For this review, take the finished solid that the model builds, in its own axes (mm). Face numbers are marked on the shaded views. A direction names the side the tool comes from. Give positions to 0.01 mm unless a question says otherwise; leave off trailing zeros. Write each loop counter-clockwise with the first axis right and the second up, starting at its lowest first coordinate (ties: lowest second). Pieces come first, ordered by that corner, then holes. Notation, with made-up numbers: M -20,1 L -10,1 A27 cw -10,29 Z; hole C 59,1 d7. An arc over 180 degrees is marked long. Write item = value, one per line.
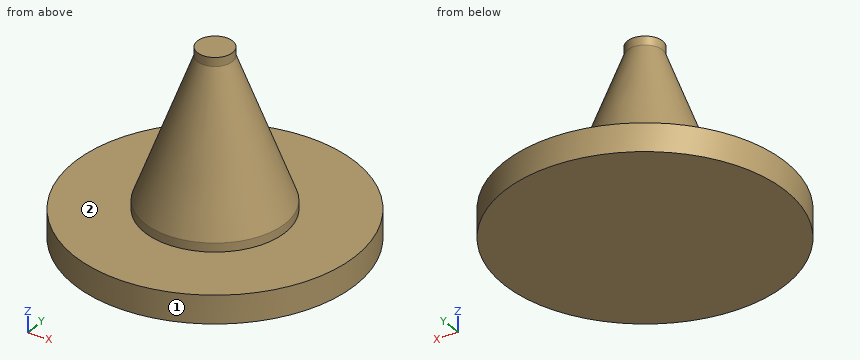
Autodesk Inventor part; units mm, degrees
ref_plane "YZ Plane" through (0, 0, 0) normal (1, 0, 0) x (0, 1, 0)
ref_plane "XZ Plane" through (0, 0, 0) normal (0, 1, 0) x (-1, 0, 0)
ref_plane "XY Plane" through (0, 0, 0) normal (0, 0, 1) x (1, 0, 0)
sketch "Sketch1" plane through (0, 0, 0) normal (0, 0, 1) x (1, 0, 0)
  circle A0 centre (0, 0) radius 12.7
  dimension "d0" = 25.4
extrude "Extrusion1" add sketch "Sketch1" along normal blind 1.5875
ref_plane "Work Plane1" through (0, 0, 26.9875) normal (0, 0, 1) x (1, 0, 0)
sketch "Sketch2" plane through (0, 0, 26.9875) normal (0, 0, 1) x (1, 0, 0)
  circle A0 centre (0, 0) radius 3.175
  dimension "d4" = 6.35
extrude "Extrusion2" add sketch "Sketch2" along normal blind 1.5875
loft "Loft1" add section 1 edges at (-12.7, 0, 1.5875) section 2 edges at (-3.175, 0, 26.9875)
sketch "Sketch3" plane through (0, 0, 0) normal (0, 0, -1) x (-1, 0, 0)
  circle A0 centre (0, 0) radius 25.4
  dimension "d11" = 50.8
extrude "Extrusion3" add sketch "Sketch3" along normal blind 5.08
sketch "Sketch5" plane through (0, 0, -5.08) normal (0, 0, -1) x (-1, 0, 0)
  point P0 (0, 0)
properties part number "Aerospike base"
1. We need section B-B, the plane z = 9. Write out the cut boundary in (x, y), then the cut area to 3 significant figures.
Responses:
outline = C 0,0 d19.84
area = 309 mm2
2. We need section A-A, the plane x = 0. Write out the cut boundary in (y, z) (1 decimal), then the cut area to 3 significant figures.
Responses:
outline = M -25.4,-5.1 L 25.4,-5.1 L 25.4,0 L 12.7,0 L 12.7,1.6 L 3.2,27 L 3.2,28.6 L -3.2,28.6 L -3.2,27 L -12.7,1.6 L -12.7,0 L -25.4,0 Z
area = 712 mm2
3. We need section D-D, the plane z = 18. Write out the cut boundary in (x, y).
Responses:
outline = C 0,0 d13.09
4. Machinability: for the marked faces 1 and 2, which of the approach directions +Z, -Z, +X, -X, +Y, -Y give a long, thin tool a straight path to every point of the face, cutting with its end or side? Answer none if there is none.
Responses:
face_1 = +Z, -Z
face_2 = +Z
5. For line 1 along Z through (x, y) = (0, -21.5); line 2 along Y through (x, z) = (-19, -2); line 3 along Y through (x, z) = (9, 2.5), list the stretches that pass through material, from the lowest coordinate up. Write a range as from..to.
Responses:
line_1 = -5.08..0
line_2 = -16.86..16.86
line_3 = -8.47..8.47
6. We need section C-C, the plane y = -17.5. Write out the cut boundary in (x, z), then the cut area to 3 significant figures.
Responses:
outline = M -18.41,-5.08 L 18.41,-5.08 L 18.41,0 L -18.41,0 Z
area = 187 mm2
7. Insertion check: P1, Ø4, axis at y = 2, z = 15.5, coming from the +X side; P2, Ø3, axis at x = 18.5, y = -11, coming from the +Z side. Each pin has a flat end and moves straight along its axis. Give the tip position at first contact, or say it passes through.
Responses:
P1 = 8.08
P2 = 0
